Build history of the part. All positions in model axes, mm. Face numbers are marked on the shaded views. A direction names the side the tool comes from. Give positions to 0.01 mm unless a question says otherwise; leave off trailing zeros. Order: outer loops, then holes, each group sorted by start corner. A loop starts at its lowest first (then second) coordinate and runs counter-clockwise, first axis right, second up. Notation, with made-up numbers: M -7,-36 L 17,-36 A24 ccw 17,-16 Z; hole C 27.5,77.25 d2. An arc over 180 degrees is marked long. One line per item, written item: value.
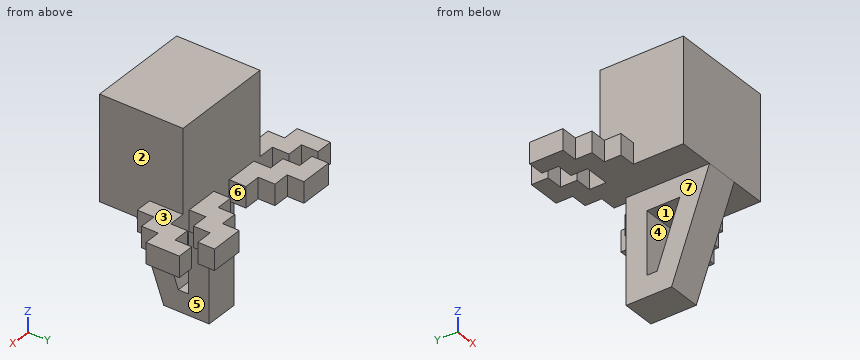
from build123d import *

# Parameters (mm, degrees)
SKETCH_1_W      = 25
SKETCH_1_H      = 20
EXTRUDE_2_DEPTH = 12.5
EXTRUDE_3_DEPTH = 4
EXTRUDE_4_DEPTH = 5


with BuildPart() as part:
    # Эскиз1 → Бобышка-Вытянуть2 (new, symmetric)
    with BuildSketch(Plane(origin=(0, 0, 0), x_dir=(0, 0, -1), z_dir=(1, 0, 0))):
        with Locations((12.5, 10)):
            Rectangle(SKETCH_1_W, SKETCH_1_H)
    extrude(amount=EXTRUDE_2_DEPTH, both=True)

    # Эскиз1<4> → Бобышка-Вытянуть3 (add, symmetric)
    with BuildSketch(Plane(origin=(0, 0, 0), x_dir=(0, 0, -1), z_dir=(1, 0, 0))):
        Polygon((25, 20), (25, 0), (50, 9.099255857), (50, 20), align=None)
        Polygon((45, 12.600293548), (30, 7.140740034), (30, 15), (45, 15), align=None, mode=Mode.SUBTRACT)
    extrude(amount=EXTRUDE_3_DEPTH, both=True)

    # Эскиз3 → Бобышка-Вытянуть4 (add)
    with BuildSketch(Plane(origin=(0, 0, -25), x_dir=(-1, 0, 0), z_dir=(0, 0, -1))):
        Polygon((-12.5, 12), (-16.5, 12), (-16.5, 16), (-20.5, 16), (-20.5, 20), (-24.5, 20), (-24.5, 28), (-20.5, 28), (-20.5, 24), (-16.5, 24), (-16.5, 20), (-12.5, 20), align=None)
        Polygon((20.5, 20), (24.5, 20), (24.5, 28), (20.5, 28), (20.5, 24), (16.5, 24), (16.5, 20), (12.5, 20), (12.5, 12), (16.5, 12), (16.5, 16), (20.5, 16), align=None)
        Polygon((-10.5, 20), (-10.5, 24), (-14.5, 24), (-14.5, 28), (-18.5, 28), (-18.5, 32), (-10.5, 32), (-10.5, 28), (-6.5, 28), (-6.5, 24), (-2.5, 24), (-2.5, 20), align=None)
        Polygon((10.5, 20), (10.5, 24), (14.5, 24), (14.5, 28), (18.5, 28), (18.5, 32), (10.5, 32), (10.5, 28), (6.5, 28), (6.5, 24), (2.5, 24), (2.5, 20), align=None)
    extrude(amount=-EXTRUDE_4_DEPTH)


solid = part.part
1) Drill centre lines: probe 1 along Y at (x, z) = (11.5, -12); probe 2 along Z at (x, y) = (7.5, 26.5); probe 3 along Z at (x, y) = (5.5, 14). Where is each one in solid material? Low to high. Write a range as from..to.
Check values:
probe 1: 0..20
probe 2: -25..-20
probe 3: -25..0
2) Pin check, flat tips, straight feed: pin 1 (2 mm diameter, centred on y = 5, z = -32.5, fed in from -X); pin 2 (4.5 mm diameter, centred on y = 31, z = -21.5, fed in from +X); pin 3 (13 mm diameter, centred on x = -16.5, y = 23, fed in from +Z); pin 4 (10 mm diameter, centred on x = 8.5, z = -5, fed in from +Y). Stop position of each tip, or through.
Check values:
pin 1: x = -4
pin 2: x = 18.5
pin 3: z = 0
pin 4: y = 20
3) Saw through at B-B, the plane x = 17.5. Write the cut outline in (y, z).
Check values:
outline: M 16,-25 L 24,-25 L 24,-20 L 16,-20 Z; M 28,-25 L 32,-25 L 32,-20 L 28,-20 Z
4) Saw through at D-D, the plane y = 25.5. Write the cut outline in (x, z), then the cut area to 3 significant figures.
Check values:
outline: M -24.5,-25 L -20.5,-25 L -20.5,-20 L -24.5,-20 Z; M -14.5,-25 L -6.5,-25 L -6.5,-20 L -14.5,-20 Z; M 6.5,-25 L 14.5,-25 L 14.5,-20 L 6.5,-20 Z; M 20.5,-25 L 24.5,-25 L 24.5,-20 L 20.5,-20 Z
area: 120 mm^2
5) Mould opens along Z. For the marked faces 1, 2 and 3 say: released by +Z, released by -Z, zero draft, split by the parting line, or undercut.
Check values:
face 1: undercut
face 2: zero draft
face 3: released by +Z
6) Saw through at A-A, the plane y = 22. Write the cut outline in (x, z), then the cut area to 3 significant figures.
Check values:
outline: M -24.5,-25 L -16.5,-25 L -16.5,-20 L -24.5,-20 Z; M -10.5,-25 L -2.5,-25 L -2.5,-20 L -10.5,-20 Z; M 2.5,-25 L 10.5,-25 L 10.5,-20 L 2.5,-20 Z; M 16.5,-25 L 24.5,-25 L 24.5,-20 L 16.5,-20 Z
area: 160 mm^2
7) Saw through at C-C, the plane z = -41.5. Write the cut outline in (x, y), then the cut area to 3 significant figures.
Check values:
outline: M -4,6.01 L 4,6.01 L 4,11.33 L -4,11.33 Z; M -4,15 L 4,15 L 4,20 L -4,20 Z
area: 82.6 mm^2
8) Tool access for the marked faces 4, 5, 6 and 7: list every direction of +Z, -Z, +X, -X, +Y, -Y with a clear straight run to the whole face (end or side of a thin tool).
Check values:
face 4: +X, -X
face 5: -Z, +X, +Y, -Y
face 6: +Z, -Z, +Y
face 7: -Z, -X, +Y, -Y
